Read the model definition and answer for the solid it produces. Units are mm, in the model's axes. Face numbers are marked on the shaded views. A direction names the side the tool comes from. Round coordinates to 2 decimals unless told otherwise and drop trailing zeros. Write each loop counter-clockwise with the first axis right and the second up, starting at its lowest first coordinate (ties: lowest second). Pieces come first, ordered by that corner, then holes.
from build123d import *

# Parameters (mm, degrees)
F0_W     = 172
F0_H     = 108
F1_DEPTH = 62
F3_W     = 162
F3_H     = 98
F4_DEPTH = 57
F2_R     = 5
F5_DEPTH = 25
F6_W     = 162
F6_H     = 5
F7_DEPTH = 25


with BuildPart() as f1:
    # F0 (on Front) → F1 (new body)
    with BuildSketch(Plane.XZ):
        with Locations((6.416367, 0.38575)):
            Rectangle(F0_W, F0_H)
    extrude(amount=F1_DEPTH)

    # F3 (on face) → F4 (cut)
    with BuildSketch(Plane(origin=(0, 0, 0), x_dir=(-1, 0, 0), z_dir=(0, 1, 0))):
        with Locations((-6.416367, 0.38575)):
            Rectangle(F3_W, F3_H)
    extrude(amount=-F4_DEPTH, mode=Mode.SUBTRACT)

    # F2 (on face) → F5 (cut)
    with BuildSketch(Plane.XY.offset(54.38575)):
        with Locations((6.416367, -31)):
            Circle(F2_R)
    extrude(amount=-F5_DEPTH, mode=Mode.SUBTRACT)

    # F6 (on face) → F7 (cut)
    with BuildSketch(Plane.XY.offset(54.38575)):
        with Locations((6.416367, -2.5)):
            Rectangle(F6_W, F6_H)
    extrude(amount=-F7_DEPTH, mode=Mode.SUBTRACT)


solid = f1.part
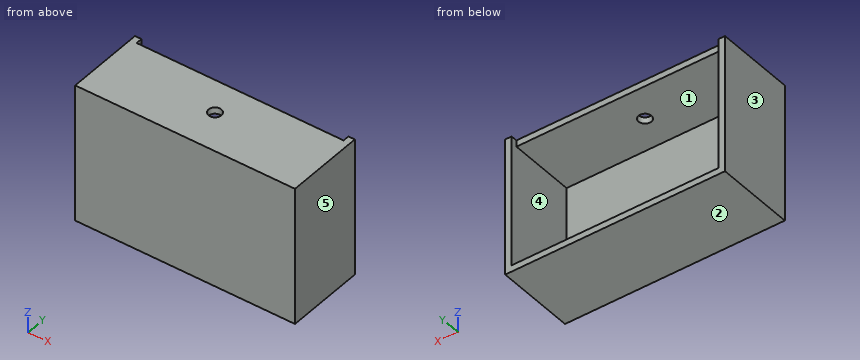
Q1. Which of the six approach directions +Z, -Z, +X, -X, +Y, -Y give full straight-line access (tool end or side, diameter ignored) to the marked faces 1 and 2?
Verdict:
face 1: +Y
face 2: -Z, +X, -X, +Y, -Y
Q2. Section D-D (x = -46) is taken. Determine the outline of the cut face in (y, z), then the cut area to 4 significant figures.
Verdict:
outline: (-62, -53.61) - (0, -53.61) - (0, -48.61) - (-57, -48.61) - (-57, 49.39) - (-5, 49.39) - (-5, 54.39) - (-62, 54.39) - close
area: 1,085 mm2
Q3. A flat-ended cylindrical pin translates along its axis: pin 1 Ø2.5 at (x, z) = (-11.5, 52) entering from +Y. Find the tip coordinate at first contact, or state that the pin passes through.
Verdict:
pin 1: stops at y = -5
Q4. Section A-A (y = -31) is taken. Determine the outline of the cut face in (x, z), then the cut area to 3 significant figures.
Verdict:
outline: (-79.58, -53.61) - (92.42, -53.61) - (92.42, 54.39) - (11.42, 54.39) - (11.42, 49.39) - (87.42, 49.39) - (87.42, -48.61) - (-74.58, -48.61) - (-74.58, 49.39) - (1.42, 49.39) - (1.42, 54.39) - (-79.58, 54.39) - close
area: 2,650 mm2
Q5. Section B-B (z = -44) is taken. Determine the outline of the cut face in (x, y), then the cut area to 3 significant figures.
Verdict:
outline: (-79.58, -62) - (92.42, -62) - (92.42, 0) - (87.42, 0) - (87.42, -57) - (-74.58, -57) - (-74.58, 0) - (-79.58, 0) - close
area: 1,430 mm2
Q6. Section C-C (y = -39.5) is taken. Determine the outline of the cut face in (x, z).
Verdict:
outline: (-79.58, -53.61) - (92.42, -53.61) - (92.42, 54.39) - (-79.58, 54.39) - close; hole (-74.58, -48.61) - (87.42, -48.61) - (87.42, 49.39) - (-74.58, 49.39) - close
Q7. Straight lines are drawn through the part: probe 1 along Z at (x, y) = (-11.5, -13.5); probe 2 along X at (y, z) = (-2.5, -6.5); probe 3 along Y at (x, z) = (-31, -40.5). For each, find the intervals that lie inside material, in ascending order.
Verdict:
probe 1: z = -53.61 to -48.61, 49.39 to 54.39
probe 2: x = -79.58 to -74.58, 87.42 to 92.42
probe 3: y = -62 to -57
Q8. Determine the mould class of the marked faces 3, 4 and 5 for opening direction X: pulls with the +X half, pulls with the -X half, needs draft (parallel to the pull), parting line crosses it, or undercut.
Verdict:
face 3: pulls with the -X half
face 4: undercut
face 5: pulls with the +X half
